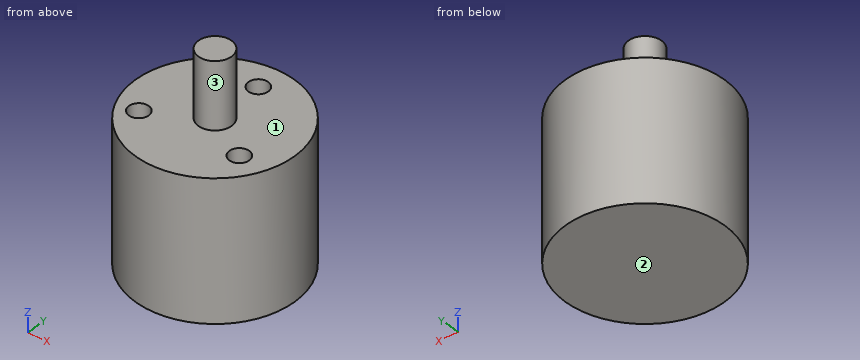
```python
from build123d import *

# Parameters (mm, degrees)
ESQUISSE1_R             = 12
BOSS_EXTRU_1_DEPTH      = 21
ESQUISSE2_R             = 2.5
BOSS_EXTRU_2_DEPTH      = 10
ESQUISSE3_R             = 1.5
ESQUISSE3_R_2           = 1.501649619
ENL_V_MAT_EXTRU_1_DEPTH = 4


with BuildPart() as part:
    # Esquisse1 → Boss.-Extru.1 (new body)
    with BuildSketch(Plane.XY):
        with Locations(Location((0, 0, 0), (0, 0, 180))):
            Circle(ESQUISSE1_R)
    extrude(amount=BOSS_EXTRU_1_DEPTH)

    # Esquisse2 → Boss.-Extru.2 (add)
    with BuildSketch(Plane.XY.offset(21)):
        Circle(ESQUISSE2_R)
    extrude(amount=BOSS_EXTRU_2_DEPTH)

    # Esquisse3 → Enlèv. mat.-Extru.1 (cut)
    with BuildSketch(Plane.XY.offset(21)):
        with Locations((0, 8)):
            Circle(ESQUISSE3_R)
        with Locations((-7.794228634, -4.5)):
            Circle(ESQUISSE3_R_2)
        with Locations((6.92820323, -4)):
            Circle(ESQUISSE3_R)
    extrude(amount=-ENL_V_MAT_EXTRU_1_DEPTH, mode=Mode.SUBTRACT)


solid = part.part
```
Here's how the part is built. I have some questions about the finished solid (model axes, mm). Face numbers are marked on the shaded views. Coordinates: 2 decimals unless noted, no trailing zeros. Order: outer loops, then holes, each group sorted by start corner. A loop starts at its lowest first (then second) coordinate and runs counter-clockwise, first axis right, second up. Notation, with made-up numbers: (30.5, -15) - (80.5, -15) arc R4 cw to (80.5, -8) - close; hole circle Ø5 at (24, -19.5). An arc over 180 degrees is marked (long way). One line per question, with ' | ' between items. Start each with the question number.
1. If we section it at C-C (z = 20): Write out the boundary of the cut face in (x, y).
2. Please list where these lines run through material, in increasing order: line 1 along Y through (x, z) = (0, 19.6); line 2 along Z through (x, y) = (-1, -7.75); line 3 along Y through (x, z) = (-7, 19). Write a range as [from, to].
3. If we section it at B-B (y = 0): Write out the boundary of the cut face in (x, z).
4. If we mould it in two halves opening along Z, with no side actions, what happens to the marked faces 1, 2 and 3? For each: released by +Z, released by -Z, zero draft, split by the parting line, or undercut.
5. If we section it at A-A (x = 0): Write out the boundary of the cut face in (y, z).
6. I'm going to push flat-ended pins straight in: pin 1 Ø5 at (x, y) = (-6, 3) entering from +Z; pin 2 Ø2.5 at (x, y) = (0, 8) entering from -Z; pin 3 Ø0.9 at (x, y) = (-8.5, -4.5) entering from +Z; pin 4 Ø6 at (y, z) = (-4, 21) entering from +X. Where does each tip first touch, or does it pass through?
7. If we section it at D-D (z = 7.5): Write out the boundary of the cut face in (x, y).
Model answer:
1) outline: circle Ø24 at (0, 0); hole circle Ø3 at (-7.79, -4.5); hole circle Ø3 at (0, 8); hole circle Ø3 at (6.93, -4)
2) line 1: y = [-12, 6.5], [9.5, 12] | line 2: z = [0, 21] | line 3: y = [-9.75, -5.77], [-3.23, 9.75]
3) outline: (-12, 0) - (12, 0) - (12, 21) - (2.5, 21) - (2.5, 31) - (-2.5, 31) - (-2.5, 21) - (-12, 21) - close
4) face 1: released by +Z | face 2: released by -Z | face 3: zero draft
5) outline: (-12, 0) - (12, 0) - (12, 21) - (9.5, 21) - (9.5, 17) - (6.5, 17) - (6.5, 21) - (2.5, 21) - (2.5, 31) - (-2.5, 31) - (-2.5, 21) - (-12, 21) - close
6) pin 1: stops at z = 21 | pin 2: stops at z = 0 | pin 3: stops at z = 17 | pin 4: stops at x = 11.96
7) outline: circle Ø24 at (0, 0)
